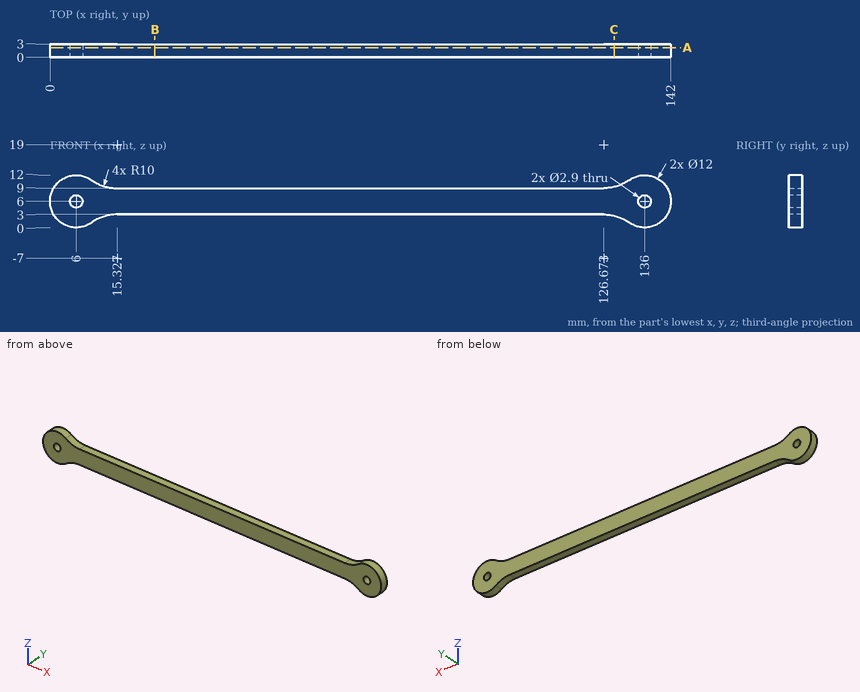
For this review, use the dimensioned drawing (mm, ordinates from the lowest corner) and the shaded views. Give positions to 0.01 mm unless a question says otherwise; leave off trailing zeros. Loops run counter-clockwise (first coordinate to the right, second up) from the corner with the lowest first, then second, coordinate; pieces in that order, holes last.
Item 1: Take a section at B-B, the plane x = 24. State the section outline as (y, z) points, and give its area (3 significant figures).
Item 2: Take a section at C-C, the plane x = 129. State the section outline as (y, z) points (1 decimal).
Item 3: For line 1 along X through (y, z) = (1.9, 6.25) (1 decimal); line 2 along Z through (x, y) = (96.5, 2.25); line 3 along X through (y, z) = (1.55, 11) (1 decimal), list the stretches that pass through material, from the lowest coordinate up.
Item 4: Take a section at A-A, the plane y = 2.15. Give the number of separate pieces and of enclosed holes in the cut face.
Item 5: Insertion check: pin 1 (1.5 mm diameter, centred on x = 102.5, z = 6, fed in from -Y); pin 2 (0.9 mm diameter, centred on x = 84.5, y = 2, fed in from -Z); pin 3 (0.9 mm diameter, centred on x = 77.5, y = 1.5, fed in from +Z). Each pin has a flat end and moves straight along its axis. Give the tip position at first contact, or say it passes through.
Calculated:
1. outline: (0, 3) - (3, 3) - (3, 9) - (0, 9) - close
1. area: 18.0 mm2
2. outline: (0, 2.7) - (3, 2.7) - (3, 9.3) - (0, 9.3) - close
3. line 1: x = 0 to 4.6, 7.4 to 134.6, 137.4 to 142
3. line 2: z = 3 to 9
3. line 3: x = 2.7 to 9.3, 132.7 to 139.3
4. separate pieces: 1
4. enclosed holes: 2
5. pin 1: stops at y = 0
5. pin 2: stops at z = 3
5. pin 3: stops at z = 9
